from build123d import *

# Parameters (mm, degrees)
SKETCH1_W           = 35
SKETCH1_H           = 35
BOSS_EXTRUDE1_DEPTH = 3
BOSS_EXTRUDE2_DEPTH = 25
CUT_EXTRUDE1_REACH  = 37.178


with BuildPart() as part:
    # Sketch1 → Boss-Extrude1 (new body)
    with BuildSketch(Plane(origin=(0, 0, 0), x_dir=(1, 0, 0), z_dir=(0, 1, 0))):
        Rectangle(SKETCH1_W, SKETCH1_H)
    extrude(amount=BOSS_EXTRUDE1_DEPTH)

    # Sketch2 → Boss-Extrude2 (add)
    with BuildSketch(Plane(origin=(0, 3, 0), x_dir=(1, 0, 0), z_dir=(0, 1, 0))):
        with BuildLine():
            Line((3.77290479, 12.126631414), (3.77290479, 15.239920913))
            ThreePointArc((3.77290479, 15.239920913), (11.101576465, -11.101576465), (-15.239920913, -3.77290479))
            Line((-15.239920913, -3.77290479), (-12.126631414, -3.77290479))
            ThreePointArc((-12.126631414, -3.77290479), (8.980256121, -8.980256121), (3.77290479, 12.126631414))
        make_face()
    extrude(amount=BOSS_EXTRUDE2_DEPTH)

    # Sketch3 → Cut-Extrude1 (cut, up to next)
    with BuildSketch(Plane(origin=(0, 3, 0), x_dir=(1, 0, 0), z_dir=(0, 1, 0)), mode=Mode.PRIVATE) as cut_extrude1_sk1:
        with BuildLine():
            Line((2.757716447, 2.757716447), (-11.984567107, 17.5))
            Line((-11.984567107, 17.5), (-17.5, 17.5))
            Line((-17.5, 17.5), (-17.5, 11.984567107))
            Line((-17.5, 11.984567107), (-2.757716447, -2.757716447))
            ThreePointArc((-2.757716447, -2.757716447), (2.757716447, -2.757716447), (2.757716447, 2.757716447))
        make_face()
    cut_extrude1_tool1 = extrude(cut_extrude1_sk1.sketch, amount=-CUT_EXTRUDE1_REACH, mode=Mode.PRIVATE) & part.part
    add(cut_extrude1_tool1.solids().sort_by_distance((-6.984587, 3, -6.984587))[0], mode=Mode.SUBTRACT)


solid = part.part
CAD build for the part. Positions are in the model's coordinates, mm. A direction names the side the tool comes from. Round coordinates to 2 decimals unless told otherwise and drop trailing zeros. Write each loop counter-clockwise with the first axis right and the second up, starting at its lowest first coordinate (ties: lowest second). Pieces come first, ordered by that corner, then holes.
(1) Slice it at D-D, the plane z = 10.5. Write the cut outline in (x, y), and give its area (3 significant figures).
(2) Slice it at B-B, the plane x = -4. Write the cut outline in (y, z).
(3) Slice it at C-C, the plane x = 12. Write the cut outline in (y, z), and give its area (3 significant figures).
(4) Slice it at A-A, the plane z = -5.5. Write the cut outline in (x, y), and give its area (3 significant figures).
(5) Mould opens along X. For faces 1 (the face through (-4.51, 1.521, -10.026)), 2 (the face through (4, 3, 4)), 3 (the face through (17.5, 1, 0)), 4 (the face through (4, 0, 4)) say: pulls with the +X half, pulls with the -X half, needs draft (parallel to the pull), parting line crosses it, or undercut.
(6) Drop flat-ended pins along their axis: P1, Ø0.9, axis at y = 12, z = -13.5, coming from the -X side; P2, Ø2, axis at y = 19, z = -9.5, coming from the +X side; P3, Ø10, axis at y = 9, z = 4.5, coming from the -X side. Give the stop position or say it passes through.
(7) 3-axis set-ups, long thin cutter, end or side, ignore diameter. For faces 5 (the face through (8.718, 15.325, 9.235)), 6 (the face through (-10.232, 1.521, -4.717)), 7 (the face through (3, 1, -17.5)), 8 (the face through (-14, 15, 3.773)): which of +Z, -Z, +X, -X, +Y, -Y reach the whole face in a straight line?
(8) Probe line 1 along Y through (x, z) = (-9.5, 8); line 2 along X through (y, z) = (12.75, 0); line 3 along Z through (x, y) = (8, 16.25). List the from-to ranges inside material, lowest first.
From the geometry:
1. outline: (-17.5, 0) - (17.5, 0) - (17.5, 3) - (11.67, 3) - (11.67, 28) - (7.14, 28) - (7.14, 3) - (-7.14, 3) - (-7.14, 28) - (-11.67, 28) - (-11.67, 3) - (-17.5, 3) - close
1. area: 331 mm2
2. outline: (0, -17.5) - (3, -17.5) - (3, -9.52) - (0, -9.52) - close; (0, 1.52) - (3, 1.52) - (3, 12.05) - (28, 12.05) - (28, 15.18) - (3, 15.18) - (3, 17.5) - (0, 17.5) - close
3. outline: (0, -17.5) - (3, -17.5) - (3, -10.12) - (28, -10.12) - (28, -4.16) - (3, -4.16) - (3, 4.16) - (28, 4.16) - (28, 10.12) - (3, 10.12) - (3, 17.5) - (0, 17.5) - close
3. area: 403 mm2
4. outline: (-17.5, 0) - (-11.02, 0) - (-11.02, 3) - (-17.5, 3) - close; (0.02, 0) - (17.5, 0) - (17.5, 3) - (14.71, 3) - (14.71, 28) - (11.45, 28) - (11.45, 3) - (0.02, 3) - close
4. area: 153 mm2
5. face 1: undercut
5. face 2: undercut
5. face 3: pulls with the +X half
5. face 4: needs draft
6. P1: stops at x = 3.77
6. P2: stops at x = 13.2
6. P3: stops at x = -15.24
7. face 5: +Y
7. face 6: +Y, -Y
7. face 7: -Z, +X, -X, +Y, -Y
7. face 8: -Z, -X, +Y
8. line 1: y = 0 to 3
8. line 2: x = 12.7 to 15.7
8. line 3: z = -13.51 to -9.86, 9.86 to 13.51
